Autodesk Inventor part; units mm, degrees
ref_plane "YZ Plane" through (0, 0, 0) normal (1, 0, 0) x (0, 1, 0)
ref_plane "XZ Plane" through (0, 0, 0) normal (0, 1, 0) x (-1, 0, 0)
ref_plane "XY Plane" through (0, 0, 0) normal (0, 0, 1) x (1, 0, 0)
sketch "Sketch1" plane through (0, 0, 0) normal (0, 0, 1) x (1, 0, 0)
  circle A0 centre (0, 0) radius 26
  circle A1 centre (0, 0) radius 5
  dimension "d0" = 52
  dimension "d1" = 10
extrude "Extrusion1" add sketch "Sketch1" along normal mid plane 5
fillet "Fillet1" radius 1.5 1 edges at (-5, 0, 2.5)
properties part number "Rubber"
The model under review builds one solid part; all positions refer to its coordinate system, in mm. Coordinates: 2 decimals unless noted, no trailing zeros. Loops run counter-clockwise (first coordinate to the right, second up) from the corner with the lowest first, then second, coordinate; pieces in that order, holes last. Notation, with made-up numbers: M 21.5,50.25 L 78.5,50.25 A7 cw 78.5,59.25 Z; hole C -32,15.25 d6. An arc over 180 degrees is marked long. Put each result on its own line as item: value. Start each with the question number.
Q1. Add section C-C (z = 0.1). Write out the cut boundary in (x, y), and give its area (3 significant figures).
Q2. The part is to be moulded in two halves that separate along X. For faces 1 (the cylindrical face through (-1.08, 4.88, -0.77)), 2 (the cylindrical face through (-20.633, 15.821, -0.035)), 3 (the flat face through (5, -5, 2.5)), say which applies: +X half, -X half, draft (parallel to the pull), parting line (faces both ways), or undercut.
Q3. Add section D-D (y = -17.5). Write out the cut boundary in (x, z), and give its area (3 significant figures).
Q4. Clearance check with flat-ended pins moving along their axes: pin 1 (1.5 mm diameter, centred on x = 7, z = 2, fed in from +Y); pin 2 (1 mm diameter, centred on x = -4.5, z = -1.5, fed in from -Y). State where each tip first meets the part, or that it passes through.
Q5. Add section A-A (y = 0). Write out the cut boundary in (x, z), and give its area (3 significant figures).
Q6. Wall thickness on line 1 (Y direction, x = 0, z = -1.8); line 2 (Y direction, x = 2, z = 0.1); line 3 (X direction, y = -2.5, z = -0.1): over which ranges is each line inside the solid? List them lowest first.
Answers:
1. outline: C 0,0 d52; hole C 0,0 d10
1. area: 2,050 mm^2
2. face 1: undercut
2. face 2: parting line
2. face 3: draft
3. outline: M -19.23,-2.5 L 19.23,-2.5 L 19.23,2.5 L -19.23,2.5 Z
3. area: 192 mm^2
4. pin 1: stops at y = 25.24
4. pin 2: stops at y = -25.69
5. outline: M -26,-2.5 L -5,-2.5 L -5,1 A1.5 ccw -6.5,2.5 L -26,2.5 Z; M 5,-2.5 L 26,-2.5 L 26,2.5 L 6.5,2.5 A1.5 ccw 5,1 Z
5. area: 209 mm^2
6. line 1: y = -26 to -5, 5 to 26
6. line 2: y = -25.92 to -4.58, 4.58 to 25.92
6. line 3: x = -25.88 to -4.33, 4.33 to 25.88
